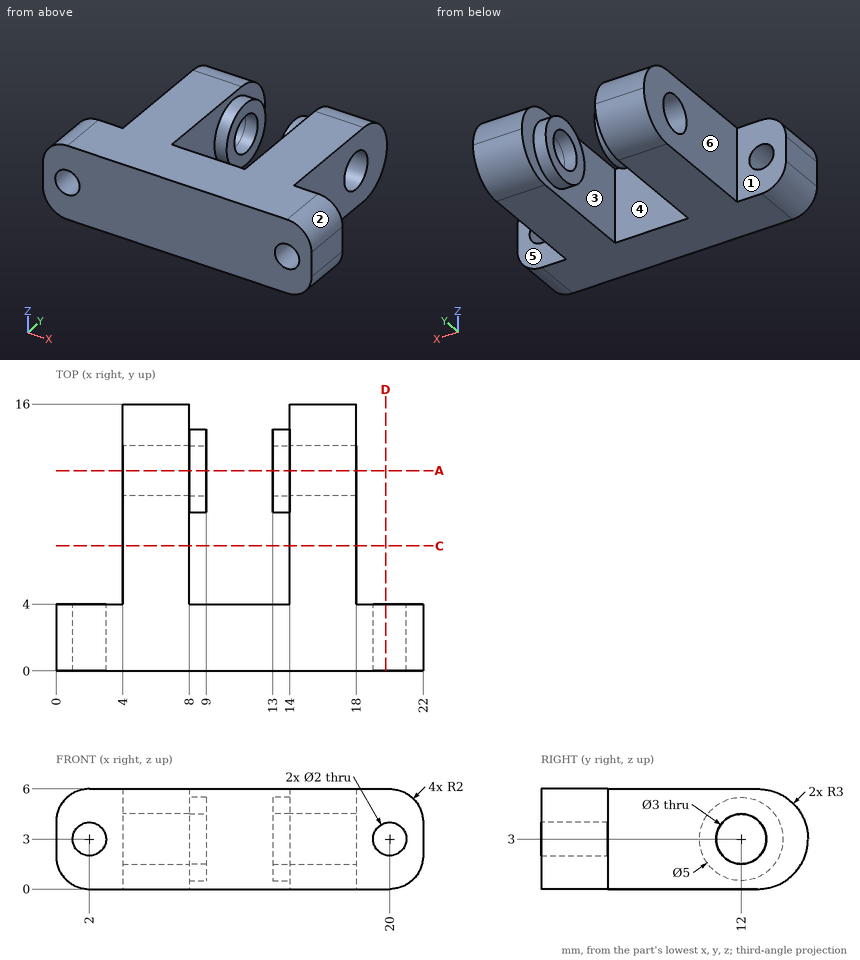
Drawing for the job (mm, zero at the part's lowest x, y, z). A direction names the side the tool comes from. Coordinates: 2 decimals unless noted, no trailing zeros. Order: outer loops, then holes, each group sorted by start corner. A loop starts at its lowest first (then second) coordinate and runs counter-clockwise, first axis right, second up.
Item 1: Two-plate mould, pull along Y, no slides. Class the marked faces 1, 2 and 3: +Y half, -Y half, draft (parallel to the pull), parting line (faces both ways), or undercut.
Check sheet entries:
face 1: +Y half
face 2: draft
face 3: undercut
Item 2: Band-saw the part on D-D on x = 19.75. List the corners of the cut face in (y, z).
Check sheet entries:
outline: (0, 0) - (4, 0) - (4, 2.03) - (0, 2.03) - close; (0, 3.97) - (4, 3.97) - (4, 6) - (0, 6) - close
Item 3: Drill centre lines: L1, parallel to Y at x = 8.65, z = 3; L2, parallel to X at y = 1.85, z = 3; L3, parallel to X at y = 14, z = 5.75. Where is each one in solid material? Low to high.
Check sheet entries:
L1: y = 0 to 4, 9.5 to 10.5, 13.5 to 14.5
L2: x = 0 to 1, 3 to 19, 21 to 22
L3: x = 4 to 8, 14 to 18
Item 4: Band-saw the part on C-C on y = 7.5. List the corners of the cut face in (x, z), plus the area to 3 significant figures.
Check sheet entries:
outline: (4, 0) - (8, 0) - (8, 6) - (4, 6) - close; (14, 0) - (18, 0) - (18, 6) - (14, 6) - close
area: 48.0 mm2
Item 5: 3-axis set-ups, long thin cutter, end or side, ignore diameter. For the marked faces 4, 5 and 6: which of +Z, -Z, +X, -X, +Y, -Y reach the whole face in a straight line?
Check sheet entries:
face 4: +Z, -Z
face 5: +Z, -Z, +X, +Y
face 6: +Z, -Z, -X, +Y
Item 6: Band-saw the part on A-A on y = 12. List the corners of the cut face in (x, z).
Check sheet entries:
outline: (4, 0) - (8, 0) - (8, 0.5) - (9, 0.5) - (9, 1.5) - (4, 1.5) - close; (4, 4.5) - (9, 4.5) - (9, 5.5) - (8, 5.5) - (8, 6) - (4, 6) - close; (13, 0.5) - (14, 0.5) - (14, 0) - (18, 0) - (18, 1.5) - (13, 1.5) - close; (13, 4.5) - (18, 4.5) - (18, 6) - (14, 6) - (14, 5.5) - (13, 5.5) - close
Item 7: Pin check, flat tips, straight feed: pin 1 Ø1.5 at (x, z) = (18.5, 4) entering from -Y; pin 2 Ø1.5 at (y, z) = (12, 2) entering from -X. Stop position of each tip, or through.
Check sheet entries:
pin 1: stops at y = 0
pin 2: stops at x = 4
